Could you check a few things on this model? Use its own coordinates, in mm. Face numbers are marked on the shaded views. Round coordinates to 2 decimals unless told otherwise and drop trailing zeros. Loops run counter-clockwise (first coordinate to the right, second up) from the corner with the lowest first, then second, coordinate; pieces in that order, holes last. Notation, with made-up numbers: (-29.75, 33.5) -> (-6.75, 33.5) arc R21 ccw to (-6.75, 41.5) -> close; hole circle Ø3 at (-9.75, 0). An arc over 180 degrees is marked (long way). One line per item, written item: value.
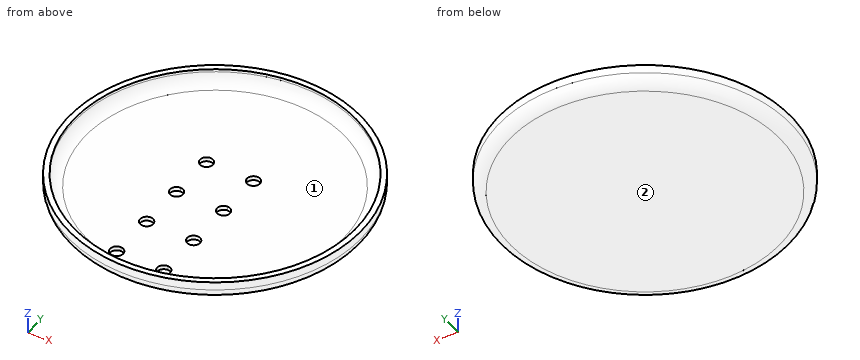
from build123d import *

# Parameters (mm, degrees)
F0_R     = 66.675
F1_DEPTH = 2.54
F2_R     = 66.675
F2_R_2   = 64.135
F3_DEPTH = 6.35
F4_R     = 5.08
F6_DEPTH = 1.9538461538


with BuildPart() as f1:
    # F0 (on Top) → F1 (new body)
    with BuildSketch(Plane.XY):
        Circle(F0_R)
    extrude(amount=F1_DEPTH)

    # F2 (on face) → F3 (join)
    with BuildSketch(Plane.XY.offset(2.54)):
        Circle(F2_R)
        Circle(F2_R_2, mode=Mode.SUBTRACT)
    extrude(amount=F3_DEPTH)

    # F4
    f4_edges = [f1.edges().sort_by_distance(p)[0] for p in [
        (-64.135, 0, 2.54),
        (-66.675, 0, 0),
    ]]
    fillet(f4_edges, radius=F4_R)

    # F5 (on face) → F6 (cut)
    with BuildSketch(Plane.XY.offset(2.54)):
        with BuildLine():
            Line((10.795, 10.795), (7.8184375, 10.795))
            ThreePointArc((7.8184375, 10.795), (8.6902524716, 8.6902524716), (10.795, 7.8184375))
            Line((10.795, 7.8184375), (10.795, 10.795))
        make_face()
        with BuildLine():
            ThreePointArc((13.7715625, 10.795), (10.795, 13.7715625), (7.8184375, 10.795))
            Line((7.8184375, 10.795), (10.795, 10.795))
            Line((10.795, 10.795), (10.795, 7.8184375))
            ThreePointArc((10.795, 7.8184375), (12.8997475284, 8.6902524716), (13.7715625, 10.795))
        make_face()
        with BuildLine():
            Line((-10.795, 10.795), (-7.8184375, 10.795))
            ThreePointArc((-7.8184375, 10.795), (-12.8997475284, 12.8997475284), (-10.795, 7.8184375))
            Line((-10.795, 7.8184375), (-10.795, 10.795))
        make_face()
        with BuildLine():
            ThreePointArc((-10.795, 7.8184375), (-8.6902524716, 8.6902524716), (-7.8184375, 10.795))
            Line((-7.8184375, 10.795), (-10.795, 10.795))
            Line((-10.795, 10.795), (-10.795, 7.8184375))
        make_face()
        with BuildLine():
            Line((10.795, -10.795), (10.795, -7.8184375))
            ThreePointArc((10.795, -7.8184375), (8.6902524716, -8.6902524716), (7.8184375, -10.795))
            Line((7.8184375, -10.795), (10.795, -10.795))
        make_face()
        with BuildLine():
            ThreePointArc((13.7715625, -10.795), (12.8997475284, -8.6902524716), (10.795, -7.8184375))
            Line((10.795, -7.8184375), (10.795, -10.795))
            Line((10.795, -10.795), (7.8184375, -10.795))
            ThreePointArc((7.8184375, -10.795), (10.795, -13.7715625), (13.7715625, -10.795))
        make_face()
        with BuildLine():
            ThreePointArc((-7.8184375, -10.795), (-8.6902524716, -8.6902524716), (-10.795, -7.8184375))
            Line((-10.795, -7.8184375), (-10.795, -10.795))
            Line((-10.795, -10.795), (-7.8184375, -10.795))
        make_face()
        with BuildLine():
            Line((-10.795, -10.795), (-10.795, -7.8184375))
            ThreePointArc((-10.795, -7.8184375), (-12.8997475284, -12.8997475284), (-7.8184375, -10.795))
            Line((-7.8184375, -10.795), (-10.795, -10.795))
        make_face()
        with BuildLine():
            Line((10.795, -32.385), (7.8184375, -32.385))
            ThreePointArc((7.8184375, -32.385), (8.6902524716, -34.4897475284), (10.795, -35.3615625))
            Line((10.795, -35.3615625), (10.795, -32.385))
        make_face()
        with BuildLine():
            ThreePointArc((13.7715625, -32.385), (10.795, -29.4084375), (7.8184375, -32.385))
            Line((7.8184375, -32.385), (10.795, -32.385))
            Line((10.795, -32.385), (10.795, -35.3615625))
            ThreePointArc((10.795, -35.3615625), (12.8997475284, -34.4897475284), (13.7715625, -32.385))
        make_face()
        with BuildLine():
            Line((-10.795, -32.385), (-7.8184375, -32.385))
            ThreePointArc((-7.8184375, -32.385), (-12.8997475284, -30.2802524716), (-10.795, -35.3615625))
            Line((-10.795, -35.3615625), (-10.795, -32.385))
        make_face()
        with BuildLine():
            ThreePointArc((-10.795, -35.3615625), (-8.6902524716, -34.4897475284), (-7.8184375, -32.385))
            Line((-7.8184375, -32.385), (-10.795, -32.385))
            Line((-10.795, -32.385), (-10.795, -35.3615625))
        make_face()
        with BuildLine():
            ThreePointArc((13.7715625, -53.975), (12.8997475284, -51.8702524716), (10.795, -50.9984375))
            Line((10.795, -50.9984375), (10.795, -53.975))
            Line((10.795, -53.975), (7.8184375, -53.975))
            ThreePointArc((7.8184375, -53.975), (10.795, -56.9515625), (13.7715625, -53.975))
        make_face()
        with BuildLine():
            Line((-10.795, -53.975), (-10.795, -50.9984375))
            ThreePointArc((-10.795, -50.9984375), (-12.8997475284, -56.0797475284), (-7.8184375, -53.975))
            Line((-7.8184375, -53.975), (-10.795, -53.975))
        make_face()
        with BuildLine():
            Line((10.795, -53.975), (10.795, -50.9984375))
            ThreePointArc((10.795, -50.9984375), (8.6902524716, -51.8702524716), (7.8184375, -53.975))
            Line((7.8184375, -53.975), (10.795, -53.975))
        make_face()
        with BuildLine():
            ThreePointArc((-7.8184375, -53.975), (-8.6902524716, -51.8702524716), (-10.795, -50.9984375))
            Line((-10.795, -50.9984375), (-10.795, -53.975))
            Line((-10.795, -53.975), (-7.8184375, -53.975))
        make_face()
    extrude(amount=-F6_DEPTH, mode=Mode.SUBTRACT)


solid = f1.part
(1) Thinking about a two-plate mould opening in X: for the marked faces 1 and 2, which applies, released by +X, released by -X, zero draft, split by the parting line, or undercut?
Recorded:
face 1: undercut
face 2: zero draft
(2) If I drill on L1, parallel to X at y = -11, z = 2; L2, parallel to X at y = 43, z = 8.25; L3, parallel to Z at x = 11.5, y = -17.5, over which ranges is the centre line in solid material (lowest first)?
Recorded:
L1: -64.71 to -13.76, -7.83 to 7.83, 13.76 to 64.71
L2: -50.96 to -47.58, 47.58 to 50.96
L3: 0 to 2.54
(3) I'm going to push flat-ended pins straight in: pin 1 Ø5 at (x, y) = (10.5, 10) entering from +Z; pin 2 Ø5.5 at (x, y) = (-10.795, -53.975) entering from +Z; pin 3 Ø1 at (y, z) = (-25, 3.5) entering from -X. Where does each tip first touch, or does it pass through?
Recorded:
pin 1: z = 2.54
pin 2: z = 0.59
pin 3: x = -61.79
(4) If we section it at A-A, the plane x = 0: Please give me the cut outline in (y, z) (3 decimals), then the cut area to 3 significant figures.
Recorded:
outline: (-66.675, 5.08) arc R5.08 ccw to (-61.595, 0) -> (61.595, 0) arc R5.08 ccw to (66.675, 5.08) -> (66.675, 8.89) -> (64.135, 8.89) -> (64.135, 7.62) arc R5.08 cw to (59.055, 2.54) -> (-59.055, 2.54) arc R5.08 cw to (-64.135, 7.62) -> (-64.135, 8.89) -> (-66.675, 8.89) -> close
area: 371 mm²
